Autodesk Inventor part; units mm, degrees
ref_plane "YZ Plane" through (0, 0, 0) normal (1, 0, 0) x (0, 1, 0)
ref_plane "XZ Plane" through (0, 0, 0) normal (0, 1, 0) x (-1, 0, 0)
ref_plane "XY Plane" through (0, 0, 0) normal (0, 0, 1) x (1, 0, 0)
sketch "Sketch1" plane through (0, 0, 0) normal (0, 0, 1) x (1, 0, 0)
  line L0 (0, 0) -> (-393.7, 0)
  line L1 (-393.7, 0) -> (-393.7, 114.3)
  line L2 (0, 203.2) -> (0, 0)
  circle A0 centre (-38.1, 114.3) radius 50.8 construction
  circle A1 centre (-38.1, 114.3) radius 6.35 construction
  circle A2 centre (-38.1, 114.3) radius 14.2875
  line L3 (-38.1, 114.3) -> (-38.1, 165.1)
  arc A3 (-384.7802, 193.4467) -> (-393.7, 114.3) centre (-38.1, 114.3) ccw
  arc A4 (-338.2351, 305.01) -> (-393.6892, 111.5268) centre (-38.1, 114.3) ccw
  circle A5 centre (-38.1, 114.3) radius 282.575 construction
  circle A6 centre (-38.1, 114.3) radius 327.025 construction
  circle A7 centre (-38.1, 114.3) radius 304.8 construction
  arc A8 (-372.5283, 214.9641) -> (-378.0555, 34.2635) centre (-38.1, 114.3) ccw
  arc A9 (-287.4011, 189.3405) -> (-291.5214, 54.6365) centre (-38.1, 114.3) ccw
  arc A10 (-287.4011, 189.3405) -> (-372.5283, 214.9641) centre (-329.9647, 202.1523) ccw construction
  arc A11 (-378.0555, 34.2635) -> (-291.5214, 54.6365) centre (-334.7884, 44.45) ccw construction
  line L4 (-38.1, 114.3) -> (-329.9647, 202.1523) construction
  line L5 (-38.1, 114.3) -> (-334.7884, 44.45) construction
  circle A12 centre (-301.445, 216.7599) radius 3.175
  circle A13 centre (-344.1211, 229.6101) radius 3.175
  circle A14 centre (-350.5965, 17.9088) radius 3.175
  circle A15 centre (-307.2148, 28.1267) radius 3.175
  line L6 (0, 203.2) -> (-338.2351, 305.01)
  point P0 (-356.4219, 39.3568)
  point P1 (-313.1549, 49.5432)
  point P2 (-308.6829, 195.7464)
  point P3 (-351.2465, 208.5582)
  point P4 (-384.7802, 193.4467)
  dimension "d2" = 101.6
  dimension "d38" = 609.6
  dimension "d3" = 12.7
  dimension "d4" = 28.575
  dimension "d5" = 114.3
  dimension "d22" = 114.3
  dimension "d24" = 38.1
  dimension "d25" = 304.8
  dimension "d30" = 565.15
  dimension "d31" = 654.05
  dimension "d39" = 30
  dimension "d40" = 88.9
  dimension "d43" = 6.35
  dimension "d44" = 6.35
  dimension "d45" = 6.35
  dimension "d46" = 6.35
  dimension "d47" = 22.225
  dimension "d48" = 22.225
  dimension "d49" = 22.225
  dimension "d50" = 22.225
  dimension "d51" = 203.2
extrude "Extrusion1" add sketch "Sketch1" along normal blind 6.35
sketch "Sketch2" plane through (0, 0, 6.35) normal (0, 0, 1) x (1, 0, 0)
  point P0 (0, 0)
sketch "Sketch3" plane through (0, 0, 6.35) normal (0, 0, 1) x (1, 0, 0)
  line L0 (0, 0) -> (0, 203.2)
  line L1 (0, 203.2) -> (-338.2351, 305.01)
  arc A0 (-338.2351, 305.01) -> (-393.7, 114.3) centre (-38.1, 114.3) ccw
  line L2 (-393.7, 114.3) -> (-393.7, 0)
  line L3 (-393.7, 0) -> (0, 0)
  circle A1 centre (-38.1, 114.3) radius 14.2875
  circle A2 centre (-350.5965, 17.9088) radius 3.175
  circle A3 centre (-307.2148, 28.1267) radius 3.175
  circle A4 centre (-344.1211, 229.6101) radius 3.175
  circle A5 centre (-301.445, 216.7599) radius 3.175
  line L4 (0, 0) -> (0, 203.2)
  line L5 (0, 159.181) -> (-359.1138, 267.2755)
  dimension "d52" = 31.75
extrude "Extrusion2" cut sketch "Sketch3" against normal blind 25.4 contours L5 A0 L1 L0
properties part number "TurretPanel"
Can you work these out from the model? Positions are in its coordinate system, mm. Round coordinates to 2 decimals unless told otherwise and drop trailing zeros. Loops run counter-clockwise (first coordinate to the right, second up) from the corner with the lowest first, then second, coordinate; pieces in that order, holes last. Notation, with made-up numbers: M -12,-9.5 L 47,-9.5 A28 ccw 47,27.5 Z; hole C -11.75,1.5 d3. An arc over 180 degrees is marked long. Write item = value, one per line. Start each with the question number.
(1) Suppose I cut it at A-A on x = -38.1. Write out the boundary of the cut face in (y, z).
(2) If we mould it in two halves opening along X, with no side actions, what happens to faces 1 (the face through (-200, 106, 6.35)), 2 (the face through (-25, 120, 3)), 3 (the face through (-391.525, 153.569, 3.131))? For each: released by +X, released by -X, zero draft, split by the parting line, or undercut.
(3) I'm going to push a flat-ended pin straight in: P1, Ø5, axis at x = -350.6, y = 17.91, coming from the -Z side. Where does the tip first touch, or does it pass through?
(4) I need wall thicknesses on line 1 along X through (y, z) = (114.5, 0.5); line 2 along X through (y, z) = (15, 1.75); line 3 along Y through (x, z) = (-31, 1.5). Which ranges of each line are inside material? Lowest first, please.
(5) Suppose I cut it at B-B on z = 2. Give the number of separate pieces and of enclosed holes in the cut face, plus the area to 3 significant figures.
(6) Suppose I cut it at C-C on y = 178. Write out the boundary of the cut face in (x, z), plus the area to 3 significant figures.
(7) Suppose I cut it at D-D on x = -275.5. Write out the boundary of the cut face in (y, z).
Answer block:
q1.outline = M 0,0 L 100.01,0 L 100.01,6.35 L 0,6.35 Z; M 128.59,0 L 170.65,0 L 170.65,6.35 L 128.59,6.35 Z
q2.face_1 = zero draft
q2.face_2 = undercut
q2.face_3 = released by -X
q3.P1 = through
q4.line_1 = -393.7 to -52.39, -23.81 to 0
q4.line_2 = -393.7 to -351.87, -349.32 to 0
q4.line_3 = 0 to 101.9, 126.7 to 168.51
q5.separate_pieces = 1
q5.enclosed_holes = 5
q5.area = 83,300 mm²
q6.outline = M -387.95,0 L -62.52,0 L -62.52,6.35 L -387.95,6.35 Z
q6.area = 2,070 mm²
q7.outline = M 0,0 L 242.11,0 L 242.11,6.35 L 0,6.35 Z
